Could you check a few things on this drawing? It's one solid part, dimensions in mm from its lowest x, y, z. Give positions to 0.01 mm unless a question says otherwise; leave off trailing zeros. Order: outer loops, then holes, each group sorted by start corner. A loop starts at its lowest first (then second) coordinate and runs counter-clockwise, first axis right, second up. Notation, with made-up numbers: (29, 68) -> (70, 68) arc R28 ccw to (70, 90) -> close; hole circle Ø2 at (-38, -24.5). An arc over 180 degrees is marked (long way). Answer as a JSON object with one key per item and string values.
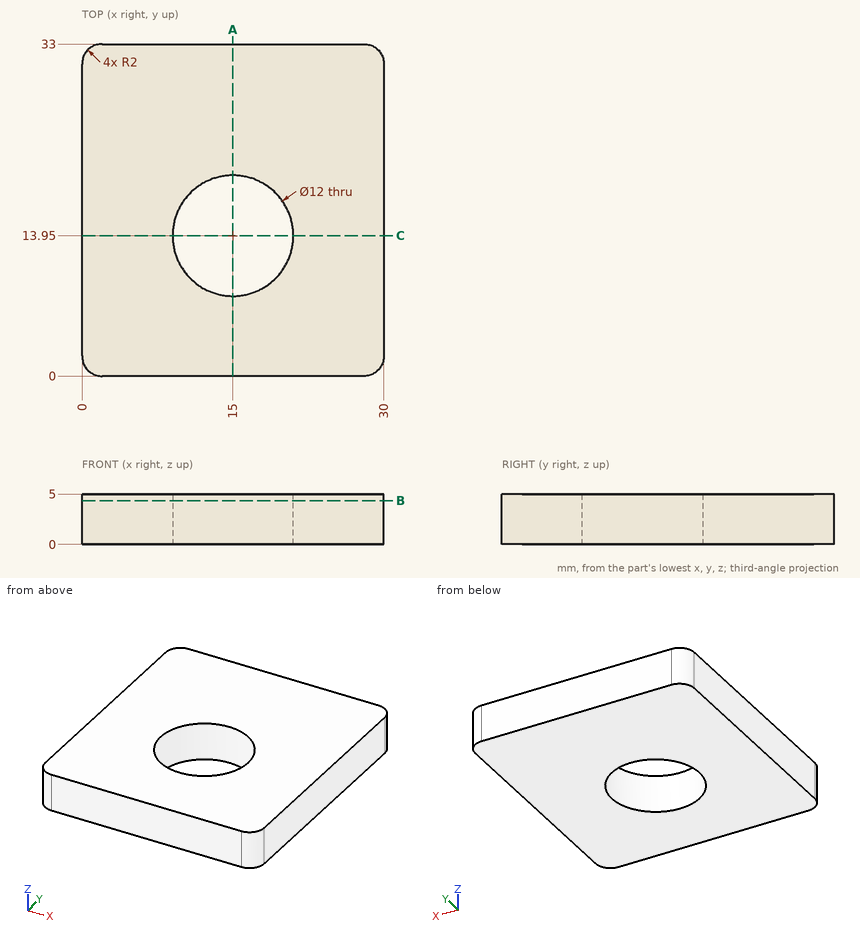
1. If we section it at A-A on x = 15: Please give me the cut outline in (y, z).
Worked answers:
{"outline": "(0, 0) -> (7.95, 0) -> (7.95, 5) -> (0, 5) -> close; (19.95, 0) -> (33, 0) -> (33, 5) -> (19.95, 5) -> close"}
2. If we section it at C-C on y = 13.95: Please give me the cut outline in (x, z), then the cut area to 3 significant figures.
Worked answers:
{"outline": "(0, 0) -> (9, 0) -> (9, 5) -> (0, 5) -> close; (21, 0) -> (30, 0) -> (30, 5) -> (21, 5) -> close", "area": "90.0 mm²"}
3. Please list where these lines run through material, in increasing order: L1, parallel to Y at x = 15, z = 2.6; L2, parallel to X at y = 11, z = 0.5; L3, parallel to X at y = 18, z = 0.3.
Worked answers:
{"L1": "0 to 7.95, 19.95 to 33", "L2": "0 to 9.78, 20.22 to 30", "L3": "0 to 10.57, 19.43 to 30"}
4. Will this pin go through, and if not, where does the flat tip stop? pin 1 Ø15.5 at (x, y) = (15, 13.95) entering from -Z.
Worked answers:
{"pin 1": "z = 0"}
5. If we section it at B-B on z = 4.35: Please give me the cut outline in (x, y), then the cut area to 3 significant figures.
Worked answers:
{"outline": "(0, 2) arc R2 ccw to (2, 0) -> (28, 0) arc R2 ccw to (30, 2) -> (30, 31) arc R2 ccw to (28, 33) -> (2, 33) arc R2 ccw to (0, 31) -> close; hole circle Ø12 at (15, 13.95)", "area": "873 mm²"}
